The listing builds one solid part. Answer for the finished solid, in the listing's coordinates (mm). Face numbers are marked on the shaded views. Round coordinates to 2 decimals unless told otherwise and drop trailing zeros. Write each loop counter-clockwise with the first axis right and the second up, starting at its lowest first coordinate (ties: lowest second). Pieces come first, ordered by that corner, then holes.
Item 1: For a pull along Z with two mould halves and no side action, classify the marked faces 1, 2, 3 and 4 as +Z half, -Z half, draft (parallel to the pull), parting line (faces both ways), or undercut.
Item 2: Find section A-A on z = -16. Give the vertices of the cut face in (x, y).
Item 3: Find section B-B on x = 24. Give the vertices of the cut face in (y, z).
Item 4: Find section C-C on y = 6. Give the vertices of the cut face in (x, z).
Item 5: Find the intervals of material crossed by probe 1 along X at (y, z) = (1.35, -16); probe 2 along Z at (x, y) = (8, 2); probe 3 along X at (y, z) = (4.75, -14), in increasing order.
Item 6: Find section D-D on y = 2.75. Give the vertices of the cut face in (x, z).
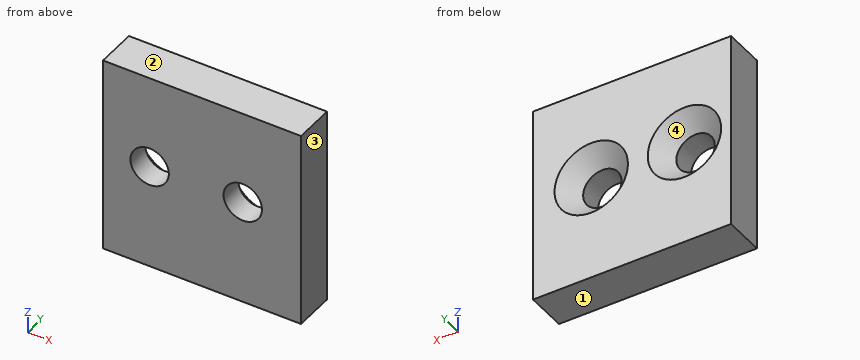
```python
from build123d import *

# Parameters (mm, degrees)
SKETCH3_W                                       = 34
SKETCH3_H                                       = 34
BOSS_EXTRUDE2_DEPTH                             = 7
CSK_FOR_M6_FLAT_HEAD_MACHINE_SCREW1_D           = 6.6
CSK_FOR_M6_FLAT_HEAD_MACHINE_SCREW1_CSINK_D     = 12.6
CSK_FOR_M6_FLAT_HEAD_MACHINE_SCREW1_CSINK_ANGLE = 90


with BuildPart() as part:
    # Sketch3 → Boss-Extrude2 (new body)
    with BuildSketch(Plane(origin=(0, 0, 0), x_dir=(1, 0, 0), z_dir=(0, 1, 0))):
        with Locations((17, 17)):
            Rectangle(SKETCH3_W, SKETCH3_H)
    extrude(amount=BOSS_EXTRUDE2_DEPTH)

    # CSK for M6 Flat Head Machine Screw1 (through all)
    with Locations(Plane(origin=(0, 7, 0), x_dir=(1, 0, 0), z_dir=(0, 1, 0))):
        with Locations((8, 16), (24, 16)):
            CounterSinkHole(CSK_FOR_M6_FLAT_HEAD_MACHINE_SCREW1_D / 2, CSK_FOR_M6_FLAT_HEAD_MACHINE_SCREW1_CSINK_D / 2, counter_sink_angle=CSK_FOR_M6_FLAT_HEAD_MACHINE_SCREW1_CSINK_ANGLE)


solid = part.part
```
Check values:
1. face 1: -Z half
1. face 2: +Z half
1. face 3: draft
1. face 4: undercut
2. outline: (0, 0) - (4.7, 0) - (4.7, 4) - (1.7, 7) - (0, 7) - close; (11.3, 0) - (20.7, 0) - (20.7, 4) - (17.7, 7) - (14.3, 7) - (11.3, 4) - close; (27.3, 0) - (34, 0) - (34, 7) - (30.3, 7) - (27.3, 4) - close
3. outline: (0, -34) - (7, -34) - (7, -22.3) - (4, -19.3) - (0, -19.3) - close; (0, -12.7) - (4, -12.7) - (7, -9.7) - (7, 0) - (0, 0) - close
4. outline: (0, -34) - (34, -34) - (34, 0) - (0, 0) - close; hole circle Ø10.6 at (8, -16); hole circle Ø10.6 at (24, -16)
5. probe 1: x = 0 to 4.7, 11.3 to 20.7, 27.3 to 34
5. probe 2: z = -34 to -19.3, -12.7 to 0
5. probe 3: x = 0 to 4.48, 11.52 to 20.48, 27.52 to 34
6. outline: (0, -34) - (34, -34) - (34, 0) - (0, 0) - close; hole circle Ø6.6 at (8, -16); hole circle Ø6.6 at (24, -16)
